Part model, mm, in its own coordinate system. Coordinates: 2 decimals unless noted, no trailing zeros. Loops run counter-clockwise (first coordinate to the right, second up) from the corner with the lowest first, then second, coordinate; pieces in that order, holes last. Notation, with made-up numbers: (86, 75.5) -> (115, 75.5) arc R17 ccw to (115, 87.5) -> close; hole circle Ø6 at (31, -12). An arc over 180 degrees is marked (long way). One line per question, with ' | ' between items. Start each with the question number.
1) Cut at C-C (x = 321). List the corners of the cut face in (y, z), plus the area to 3 significant figures.
2) Cut at B-B (y = -105.5). List the corners of the cut face in (x, z).
3) Drop flat-ended pins along their axis: pin 1 (1 mm diameter, centred on x = 1.5, z = -1, fed in from +Y); pin 2 (1.6 mm diameter, centred on y = -89, z = 0.5, fed in from -X). Give the stop position or say it passes through.
4) Cut at A-A (z = 0.3). List the corners of the cut face in (x, y), plus the area to 3 significant figures.
5) Probe L1, parallel to Y at x = 115, z = 0.35; L2, parallel to Y at x = 244, z = 0.7. List the from-to ranges inside material, lowest first. Write a range as from..to.
6) Cut at D-D (x = 408). List the corners of the cut face in (y, z), plus the area to 3 significant figures.
from build123d import *

# Parameters (mm, degrees)
BOSS_EXTRUDE1_DEPTH = 1.5875


with BuildPart() as part:
    # Sketch1 → Boss-Extrude1 (new, symmetric)
    with BuildSketch(Plane.XY):
        with BuildLine():
            Line((0, -90.664621669), (3.302, -90.664621669))
            Line((3.302, -90.664621669), (3.302, -83.806621669))
            Line((3.302, -83.806621669), (15.24, -88.786627106))
            ThreePointArc((15.24, -88.786627106), (52.629116117, -104.606478128), (92.329, -113.099587694))
            Line((92.329, -113.099587694), (92.329, -121.078455555))
            Line((92.329, -121.078455555), (95.631, -121.078455555))
            Line((95.631, -121.078455555), (95.631, -113.458455555))
            ThreePointArc((95.631, -113.458455555), (96.315178786, -113.526351883), (96.999571645, -113.59205528))
            ThreePointArc((96.999571645, -113.59205528), (143.916391113, -117.292313455), (190.924914267, -119.545890704))
            Line((190.924914267, -119.545890704), (191.088010164, -127.337201025))
            Line((191.088010164, -127.337201025), (194.389286946, -127.268095229))
            Line((194.389286946, -127.268095229), (194.229812033, -119.649764195))
            ThreePointArc((194.229812033, -119.649764195), (242.008318885, -120.352184929), (289.785425963, -119.560256171))
            Line((289.785425963, -119.560256171), (290.131623743, -127.604610112))
            Line((290.131623743, -127.604610112), (293.430570154, -127.462636259))
            Line((293.430570154, -127.462636259), (293.085752086, -119.450341713))
            ThreePointArc((293.085752086, -119.450341713), (430.886485092, -108.454741771), (567.129437002, -85.049543851))
            Line((567.129437002, -85.049543851), (582.192517176, -82.415688618))
            Line((582.192517176, -82.415688618), (583.522459193, -97.003520311))
            ThreePointArc((583.522459193, -97.003520311), (340.810991625, -132.334178874), (95.5675, -128.764621669))
            ThreePointArc((95.5675, -128.764621669), (46.062902856, -118.505679901), (0, -97.669173356))
            Line((0, -97.669173356), (0, -90.664621669))
        make_face()
    extrude(amount=BOSS_EXTRUDE1_DEPTH, both=True)


solid = part.part
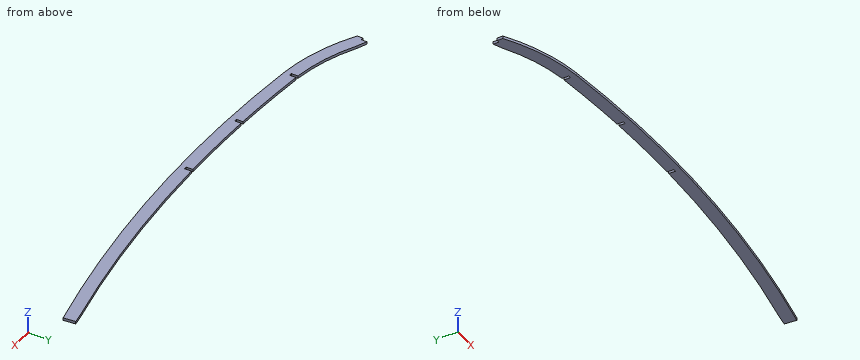
Reported:
1) outline: (-133.5, -1.59) -> (-118.23, -1.59) -> (-118.23, 1.59) -> (-133.5, 1.59) -> close | area: 48.5 mm²
2) outline: (14.35, -1.59) -> (55.53, -1.59) -> (55.53, 1.59) -> (14.35, 1.59) -> close; (453.1, -1.59) -> (543.85, -1.59) -> (543.85, 1.59) -> (453.1, 1.59) -> close
3) pin 1: stops at y = -90.66 | pin 2: stops at x = 3.3
4) outline: (0, -97.67) arc R229.78 ccw to (95.57, -128.76) arc R1543.18 ccw to (583.52, -97) -> (582.19, -82.42) -> (567.13, -85.05) arc R1527.94 cw to (293.09, -119.45) -> (293.43, -127.46) -> (290.13, -127.6) -> (289.79, -119.56) arc R1527.94 cw to (194.23, -119.65) -> (194.39, -127.27) -> (191.09, -127.34) -> (190.92, -119.55) arc R1527.94 cw to (97, -113.59) arc R214.54 cw to (95.63, -113.46) -> (95.63, -121.08) -> (92.33, -121.08) -> (92.33, -113.1) arc R214.54 cw to (15.24, -88.79) -> (3.3, -83.81) -> (3.3, -90.66) -> (0, -90.66) -> close | area: 8,900 mm²
5) L1: y = -130.47..-115.18 | L2: y = -135.59..-120.35
6) outline: (-126.48, -1.59) -> (-111.15, -1.59) -> (-111.15, 1.59) -> (-126.48, 1.59) -> close | area: 48.7 mm²
